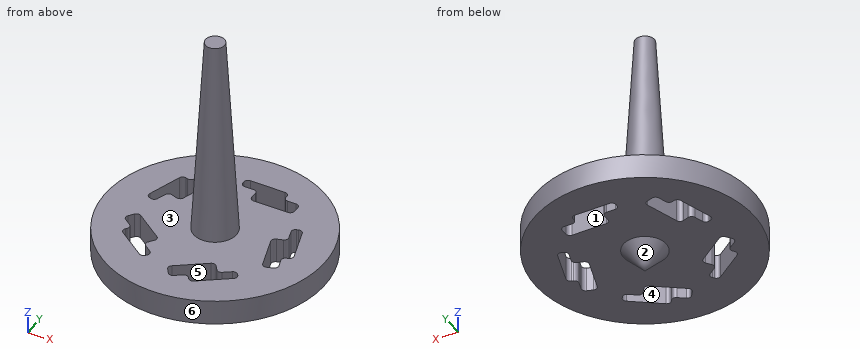
from build123d import *

# Parameters (mm, degrees)
F3_DEPTH = 7.164216


with BuildPart() as f1:
    # F0 (on Front) → F1 (revolve)
    with BuildSketch(Plane.XZ):
        Polygon((0, 38.1), (0, 0), (3.270783, 3.380191), (16.757639, 3.380191), (16.757639, 7.163216), (3.270783, 7.163216), (1.456713, 38.1), align=None)
    revolve(axis=Axis((0, 0, 19.05), (0, 0, 1)))

    # F2 (on face) → F3 (cut, through all)
    with BuildSketch(Plane.XY.offset(7.163216)):
        with BuildLine():
            Line((4.169526, 11.737372), (-1.219378, 11.737372))
            ThreePointArc((-1.219378, 11.737372), (-1.668391, 11.551385), (-1.854378, 11.102372))
            Line((-1.854378, 11.102372), (-1.854378, 10.813008))
            ThreePointArc((-1.854378, 10.813008), (-1.668391, 10.363995), (-1.219378, 10.178008))
            Line((-1.219378, 10.178008), (0.165754, 10.178008))
            ThreePointArc((0.165754, 10.178008), (0.614767, 9.992021), (0.800754, 9.543008))
            Line((0.800754, 9.543008), (0.800754, 8.579325))
            ThreePointArc((0.800754, 8.579325), (0.986741, 8.130312), (1.435754, 7.944325))
            Line((1.435754, 7.944325), (6.740368, 7.944325))
            ThreePointArc((6.740368, 7.944325), (7.189381, 8.130312), (7.375368, 8.579325))
            Line((7.375368, 8.579325), (7.375368, 9.543008))
            ThreePointArc((7.375368, 9.543008), (7.189381, 9.992021), (6.740368, 10.178008))
            Line((6.740368, 10.178008), (5.439526, 10.178008))
            ThreePointArc((5.439526, 10.178008), (4.990513, 10.363995), (4.804526, 10.813008))
            Line((4.804526, 10.813008), (4.804526, 11.102372))
            ThreePointArc((4.804526, 11.102372), (4.618538, 11.551385), (4.169526, 11.737372))
        make_face()
        with BuildLine():
            Line((-9.87445, 7.592502), (-11.539712, 2.46735))
            ThreePointArc((-11.539712, 2.46735), (-11.501581, 1.98284), (-11.132017, 1.667203))
            Line((-11.132017, 1.667203), (-10.856816, 1.577785))
            ThreePointArc((-10.856816, 1.577785), (-10.372306, 1.615917), (-10.05667, 1.98548))
            Line((-10.05667, 1.98548), (-9.62864, 3.302819))
            ThreePointArc((-9.62864, 3.302819), (-9.313003, 3.672382), (-8.828493, 3.710514))
            Line((-8.828493, 3.710514), (-7.911976, 3.41272))
            ThreePointArc((-7.911976, 3.41272), (-7.427467, 3.450851), (-7.11183, 3.820415))
            Line((-7.11183, 3.820415), (-5.472614, 8.865403))
            ThreePointArc((-5.472614, 8.865403), (-5.510745, 9.349912), (-5.880309, 9.665549))
            Line((-5.880309, 9.665549), (-6.796826, 9.963344))
            ThreePointArc((-6.796826, 9.963344), (-7.281336, 9.925212), (-7.596973, 9.555649))
            Line((-7.596973, 9.555649), (-7.998955, 8.318474))
            ThreePointArc((-7.998955, 8.318474), (-8.314592, 7.94891), (-8.799102, 7.910779))
            Line((-8.799102, 7.910779), (-9.074303, 8.000197))
            ThreePointArc((-9.074303, 8.000197), (-9.558813, 7.962065), (-9.87445, 7.592502))
        make_face()
        with BuildLine():
            Line((-10.272271, -7.044948), (-5.912556, -10.212466))
            ThreePointArc((-5.912556, -10.212466), (-5.439977, -10.325922), (-5.025587, -10.071984))
            Line((-5.025587, -10.071984), (-4.855503, -9.837883))
            ThreePointArc((-4.855503, -9.837883), (-4.742047, -9.365304), (-4.995985, -8.950914))
            Line((-4.995985, -8.950914), (-6.116581, -8.136754))
            ThreePointArc((-6.116581, -8.136754), (-6.37052, -7.722364), (-6.257063, -7.249784))
            Line((-6.257063, -7.249784), (-5.690624, -6.470148))
            ThreePointArc((-5.690624, -6.470148), (-5.577168, -5.997569), (-5.831107, -5.583179))
            Line((-5.831107, -5.583179), (-10.12263, -2.465205))
            ThreePointArc((-10.12263, -2.465205), (-10.595209, -2.351748), (-11.009599, -2.605687))
            Line((-11.009599, -2.605687), (-11.576038, -3.385323))
            ThreePointArc((-11.576038, -3.385323), (-11.689494, -3.857902), (-11.435556, -4.272292))
            Line((-11.435556, -4.272292), (-10.383152, -5.036909))
            ThreePointArc((-10.383152, -5.036909), (-10.129213, -5.451299), (-10.24267, -5.923878))
            Line((-10.24267, -5.923878), (-10.412753, -6.157978))
            ThreePointArc((-10.412753, -6.157978), (-10.52621, -6.630558), (-10.272271, -7.044948))
        make_face()
        with BuildLine():
            Line((3.525837, -11.946519), (7.885552, -8.779001))
            ThreePointArc((7.885552, -8.779001), (8.13949, -8.364611), (8.026034, -7.892031))
            Line((8.026034, -7.892031), (7.85595, -7.657931))
            ThreePointArc((7.85595, -7.657931), (7.44156, -7.403993), (6.968981, -7.517449))
            Line((6.968981, -7.517449), (5.848385, -8.331609))
            ThreePointArc((5.848385, -8.331609), (5.375806, -8.445066), (4.961416, -8.191127))
            Line((4.961416, -8.191127), (4.394977, -7.411491))
            ThreePointArc((4.394977, -7.411491), (3.980587, -7.157553), (3.508007, -7.271009))
            Line((3.508007, -7.271009), (-0.783516, -10.388983))
            ThreePointArc((-0.783516, -10.388983), (-1.037454, -10.803373), (-0.923998, -11.275952))
            Line((-0.923998, -11.275952), (-0.357559, -12.055589))
            ThreePointArc((-0.357559, -12.055589), (0.056831, -12.309527), (0.52941, -12.196071))
            Line((0.52941, -12.196071), (1.581814, -11.431454))
            ThreePointArc((1.581814, -11.431454), (2.054394, -11.317998), (2.468784, -11.571937))
            Line((2.468784, -11.571937), (2.638868, -11.806037))
            ThreePointArc((2.638868, -11.806037), (3.053258, -12.059975), (3.525837, -11.946519))
        make_face()
        with BuildLine():
            Line((12.451358, -0.338407), (10.786095, 4.786745))
            ThreePointArc((10.786095, 4.786745), (10.470458, 5.156308), (9.985949, 5.19444))
            Line((9.985949, 5.19444), (9.710747, 5.105022))
            ThreePointArc((9.710747, 5.105022), (9.341184, 4.789385), (9.303052, 4.304875))
            Line((9.303052, 4.304875), (9.731082, 2.987536))
            ThreePointArc((9.731082, 2.987536), (9.69295, 2.503026), (9.323387, 2.187389))
            Line((9.323387, 2.187389), (8.40687, 1.889595))
            ThreePointArc((8.40687, 1.889595), (8.037306, 1.573958), (7.999175, 1.089448))
            Line((7.999175, 1.089448), (9.63839, -3.95554))
            ThreePointArc((9.63839, -3.95554), (9.954027, -4.325103), (10.438537, -4.363235))
            Line((10.438537, -4.363235), (11.355054, -4.06544))
            ThreePointArc((11.355054, -4.06544), (11.724618, -3.749804), (11.762749, -3.265294))
            Line((11.762749, -3.265294), (11.360767, -2.028119))
            ThreePointArc((11.360767, -2.028119), (11.398899, -1.543609), (11.768462, -1.227972))
            Line((11.768462, -1.227972), (12.043663, -1.138554))
            ThreePointArc((12.043663, -1.138554), (12.413226, -0.822917), (12.451358, -0.338407))
        make_face()
    extrude(amount=-F3_DEPTH, mode=Mode.SUBTRACT)


solid = f1.part
Model file for the job. Use its own axes, mm. Face numbers are marked on the shaded views. A direction names the side the tool comes from. Coordinates: 2 decimals unless noted, no trailing zeros. Order: outer loops, then holes, each group sorted by start corner. A loop starts at its lowest first (then second) coordinate and runs counter-clockwise, first axis right, second up. Notation, with made-up numbers: (45, -37) -> (53, -37) arc R29 ccw to (53, 2) -> close; hole circle Ø3 at (9, -8). An arc over 180 degrees is marked (long way). Return JSON: item names as keys, results as strings. Group by question number.
Item 1: Flat gauge pins, fed straight in: P1, Ø1, axis at x = 6, z = 5, coming from the -Y side; P2, Ø0.5, axis at y = 9.5, z = 5.5, coming from the +X side; P3, Ø0.5, axis at y = 9, z = 5.5, coming from the -X side. Where does each tip first touch, or does it go through?
Item 2: Saw through at C-C on y = -13.5. Write the cut outline in (x, z), then the cut area to 3 significant figures.
Item 3: Saw through at B-B on z = 5.5. State how many separate pieces and enclosed holes the cut face has, then the cut area to 3 significant figures.
Item 4: Saw through at D-D on z = 17.5. Write the cut outline in (x, y), then the cut area to 3 significant figures.
Item 5: Pull direction Y, two halves, no side cores. Call the marked faces 3, 4, 5 and 6: pulls with the +Y half, pulls with the -Y half, needs draft (parallel to the pull), parting line crosses it, or undercut.
Item 6: Saw through at A-A on y = 6.5. Write the cut outline in (x, z), then the cut area to 3 significant figures.
Item 7: Wall check: line 1 along Z through (x, y) = (1.5, 15.5); line 2 along Y through (x, z) = (5, 4); line 3 along Y through (x, z) = (1, 26.5). Give the ranges that are in metal, low to high. Write a range as [from, to].
Item 8: Tool access for the marked faces 1 and 2: list every direction of +Z, -Z, +X, -X, +Y, -Y with a clear straight run to the whole face (end or side of a thin tool).
Values found:
{
 "1": {"P1": "stops at y = -15.83", "P2": "stops at x = 13.97", "P3": "stops at x = -14.29"},
 "2": {"outline": "(-9.93, 3.38) -> (9.93, 3.38) -> (9.93, 7.16) -> (-9.93, 7.16) -> close", "area": "75.1 mm2"},
 "3": {"separate pieces": "1", "enclosed holes": "5", "area": "759 mm2"},
 "4": {"outline": "circle Ø5.33 at (0, 0)", "area": "22.3 mm2"},
 "5": {"face 3": "needs draft", "face 4": "undercut", "face 5": "undercut", "face 6": "parting line crosses it"},
 "6": {"outline": "(-15.45, 3.38) -> (-10.23, 3.38) -> (-10.23, 7.16) -> (-15.45, 7.16) -> close; (-6.24, 3.38) -> (15.45, 3.38) -> (15.45, 7.16) -> (-6.24, 7.16) -> close", "area": "102 mm2"},
 "7": {"line 1": "z = [3.38, 7.16]", "line 2": "y = [-15.99, -10.88], [-8.24, 7.94], [10.35, 15.99]", "line 3": "y = [-1.89, 1.89]"},
 "8": {"face 1": "+Z, -Z", "face 2": "-Z"}
}
